Input: dimensioned drawing with shaded views. Units: mm. Origin: part minimum x, y, z. Coordinates: 2 decimals unless noted, no trailing zeros. Order: outer loops, then holes, each group sorted by start corner. A loop starts at its lowest first (then second) coordinate and runs counter-clockwise, first axis right, second up. Notation, with made-up numbers: (-27.75, -11) -> (17.25, -11) arc R3 ccw to (17.25, -6) -> close; hole circle Ø4 at (76.25, 0). An arc over 180 degrees is marked (long way). Write item = value, one per line. Start each with the question number.
Item 1: Section query A-A (y = 7). Output: boundary loops of the cut face in (x, z).
Item 2: Contact query for flat-ended pins moving along their axis: pin 1 (3 mm diameter, centred on x = 50.75, y = 7, fed in from -Z); pin 2 (1.2 mm diameter, centred on y = 41.5, z = 2, fed in from +X); pin 3 (1 mm diameter, centred on y = 36.5, z = 2.5, fed in from -X). Output: stop coordinate, or through.
Item 3: Mould query, pull axis X, two halves, no side actions, for the marked faces 1, 2, 3 and 4. Classes: released by +X, released by -X, zero draft, split by the parting line, or undercut.
Item 4: Section query D-D (y = 60). Output: boundary loops of the cut face in (x, z).
Item 5: Section query B-B (z = 2.4). Count the separate pieces of the cut face and the enclosed holes in it, then the cut area to 3 significant figures.
Item 6: Section query C-C (x = 7.5). Output: boundary loops of the cut face in (y, z), then the cut area to 3 significant figures.
Item 7: Ray query, line 1 along Y through (x, z) = (30, 1.2); line 2 along Y through (x, z) = (29.5, 1.35) (1 decimal); line 3 along X through (y, z) = (47, 2.4). Return the intervals inside material, ascending. Write a range as [from, to].
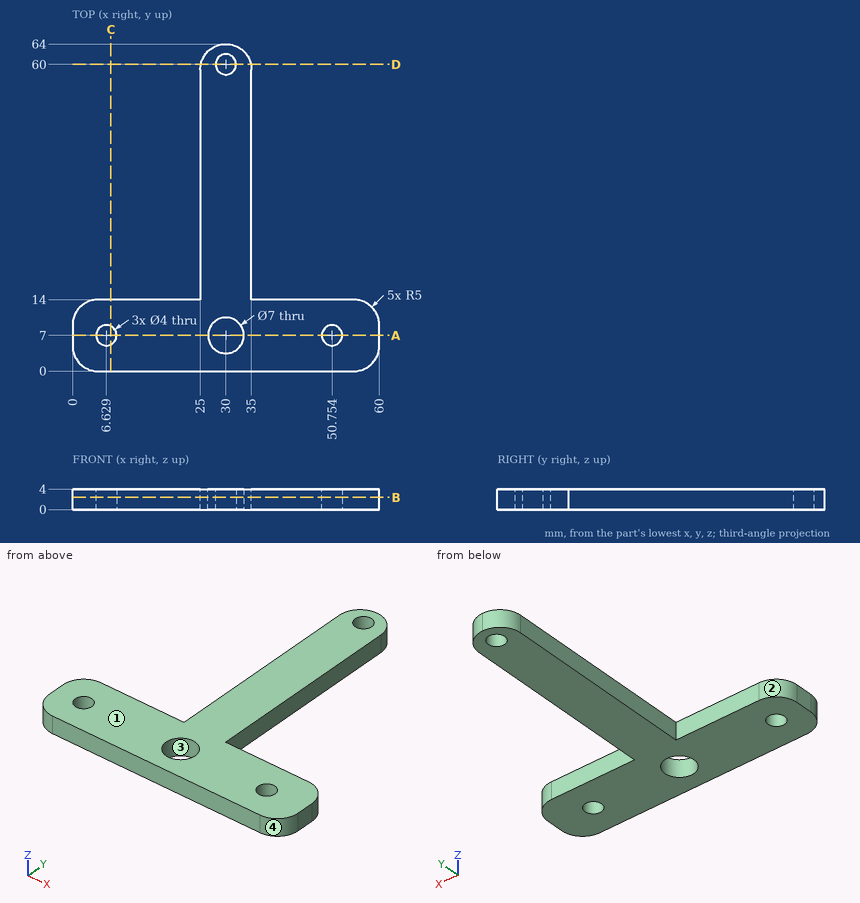
Computed:
q1.outline = (0, 0) -> (4.63, 0) -> (4.63, 4) -> (0, 4) -> close; (8.63, 0) -> (26.5, 0) -> (26.5, 4) -> (8.63, 4) -> close; (33.5, 0) -> (48.75, 0) -> (48.75, 4) -> (33.5, 4) -> close; (52.75, 0) -> (60, 0) -> (60, 4) -> (52.75, 4) -> close
q2.pin_1 = through
q2.pin_2 = 35
q2.pin_3 = 25
q3.face_1 = zero draft
q3.face_2 = released by -X
q3.face_3 = undercut
q3.face_4 = released by +X
q4.outline = (25.1, 0) -> (28, 0) -> (28, 4) -> (25.1, 4) -> close; (32, 0) -> (34.9, 0) -> (34.9, 4) -> (32, 4) -> close
q5.separate_pieces = 1
q5.enclosed_holes = 4
q5.area = 1,230 mm^2
q6.outline = (0, 0) -> (5.2, 0) -> (5.2, 4) -> (0, 4) -> close; (8.8, 0) -> (14, 0) -> (14, 4) -> (8.8, 4) -> close
q6.area = 41.6 mm^2
q7.line_1 = [0, 3.5], [10.5, 58], [62, 64]
q7.line_2 = [0, 3.5], [10.5, 58.1], [61.9, 64]
q7.line_3 = [25, 35]
